The drawing under review shows one solid part. Ordinate dimensions are in mm from its lowest x, y, z. A direction names the side the tool comes from. Round coordinates to 2 decimals unless told otherwise and drop trailing zeros. Loops run counter-clockwise (first coordinate to the right, second up) from the corner with the lowest first, then second, coordinate; pieces in that order, holes last. Notation, with made-up numbers: (41.25, 66.5) -> (54.25, 66.5) arc R35 ccw to (54.25, 102.5) -> close; hole circle Ø7 at (58.25, 6). An arc over 180 degrees is marked (long way). Use a Markdown table: item, result. Add a question column.
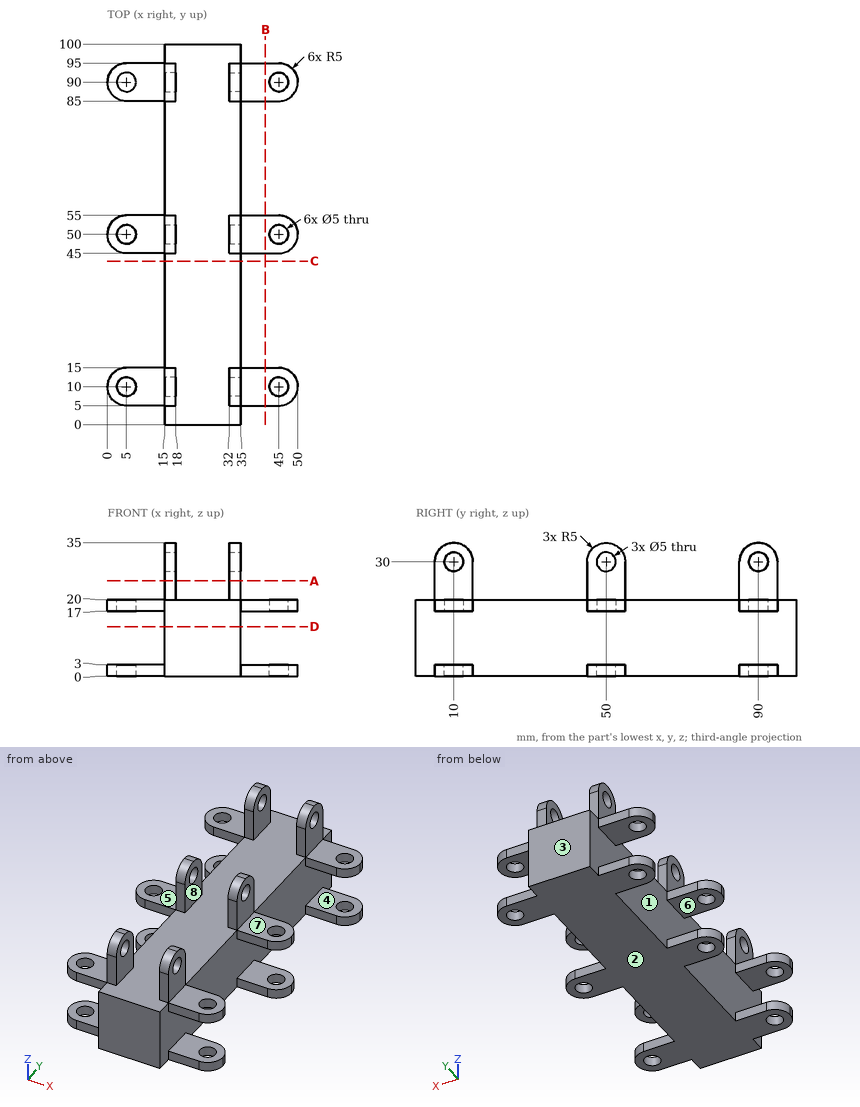
1. Mouldability with a two-part tool opening along Z and no side actions: class the marked faces 1, 2 and 3 as +Z half, -Z half, draft (parallel to the pull), parting line (faces both ways), or undercut.
2. Insertion check: P1, Ø10, axis at x = 43.5, z = 29.5, coming from the -Y side; P2, Ø0.9, axis at x = 40.5, z = 1, coming from the -Y side; P3, Ø3, axis at y = 9, z = 28, coming from the -X side; P4, Ø3.5, axis at x = 11, z = 2, coming from the +Y side. Each pin has a flat end and moves straight along its axis. Give the tip position at first contact, or say it passes through.
3. Consider section A-A on z = 25. State the section outline as (x, y) points.
4. To check wall thickness, follow probe 1 along Y at (x, z) = (5, 1.25); probe 2 along X at (y, z) = (90, 18.6); probe 3 along X at (y, z) = (45.5, 29.5). State the ranges of each line that lie inside material, in increasing order. Write a range as from..to.
5. Consider section C-C on y = 43. State the section outline as (x, z) points.
6. For the marked faces 4, 5, 6, 7 and 8, list the 3-axis set-ups (+Z, -Z, +X, -X, +Y, -Y) from which the entire face can be reached by the end or side of a thin tool; tool diameter is ignored.
7. Consider section B-B on x = 41.5. State the section outline as (y, z) points.
8. Consider section D-D on z = 13. State the section outline as (x, y) points.
Verdict:
| question | item | result |
|---|---|---|
| 1 | face 1 | undercut |
| 1 | face 2 | -Z half |
| 1 | face 3 | draft |
| 2 | P1 | passes through |
| 2 | P2 | stops at y = 5 |
| 2 | P3 | stops at x = 15 |
| 2 | P4 | stops at y = 95 |
| 3 | outline | (15, 5) -> (18, 5) -> (18, 15) -> (15, 15) -> close; (15, 45) -> (18, 45) -> (18, 55) -> (15, 55) -> close; (15, 85) -> (18, 85) -> (18, 95) -> (15, 95) -> close; (32, 5) -> (35, 5) -> (35, 15) -> (32, 15) -> close; (32, 45) -> (35, 45) -> (35, 55) -> (32, 55) -> close; (32, 85) -> (35, 85) -> (35, 95) -> (32, 95) -> close |
| 4 | probe 1 | y = 5..7.5, 12.5..15, 45..47.5, 52.5..55, 85..87.5, 92.5..95 |
| 4 | probe 2 | x = 0..2.5, 7.5..42.5, 47.5..50 |
| 4 | probe 3 | x = 15..18, 32..35 |
| 5 | outline | (15, 0) -> (35, 0) -> (35, 20) -> (15, 20) -> close |
| 6 | face 4 | +X, +Y, -Y |
| 6 | face 5 | +Z, -X, +Y, -Y |
| 6 | face 6 | -X, +Y, -Y |
| 6 | face 7 | +Z, +X, +Y, -Y |
| 6 | face 8 | +Z, +Y, -Y |
| 7 | outline | (5, 0) -> (15, 0) -> (15, 3) -> (5, 3) -> close; (5, 17) -> (15, 17) -> (15, 20) -> (5, 20) -> close; (45, 0) -> (55, 0) -> (55, 3) -> (45, 3) -> close; (45, 17) -> (55, 17) -> (55, 20) -> (45, 20) -> close; (85, 0) -> (95, 0) -> (95, 3) -> (85, 3) -> close; (85, 17) -> (95, 17) -> (95, 20) -> (85, 20) -> close |
| 8 | outline | (15, 0) -> (35, 0) -> (35, 100) -> (15, 100) -> close |
